Autodesk Inventor part; units mm, degrees
ref_plane "YZ Plane" through (0, 0, 0) normal (1, 0, 0) x (0, 1, 0)
ref_plane "XZ Plane" through (0, 0, 0) normal (0, 1, 0) x (-1, 0, 0)
ref_plane "XY Plane" through (0, 0, 0) normal (0, 0, 1) x (1, 0, 0)
sketch "Sketch1" plane through (0, 0, 0) normal (0, 1, 0) x (-1, 0, 0)
  circle A0 centre (0, 0) radius 4
  line L0 (4, 0) -> (5, 0) construction
  line L1 (5, 0) -> (5, -0.5)
  line L2 (5, -0.5) -> (3.8219, -1.1802)
  line L3 (5, 0) -> (5, 0.5)
  line L4 (5, 0.5) -> (3.8219, 1.1802)
  line L5 (3.8891, 3.182) -> (3.537, 1.868)
  line L6 (3.5355, 3.5355) -> (3.8891, 3.182)
  line L7 (3.5355, 3.5355) -> (3.182, 3.8891)
  line L8 (3.182, 3.8891) -> (1.868, 3.537)
  line L9 (0.5, 5) -> (1.1802, 3.8219)
  line L10 (0, 5) -> (0.5, 5)
  line L11 (0, 5) -> (-0.5, 5)
  line L12 (-0.5, 5) -> (-1.1802, 3.8219)
  line L13 (-3.182, 3.8891) -> (-1.868, 3.537)
  line L14 (-3.5355, 3.5355) -> (-3.182, 3.8891)
  line L15 (-3.5355, 3.5355) -> (-3.8891, 3.182)
  line L16 (-3.8891, 3.182) -> (-3.537, 1.868)
  line L17 (-5, 0.5) -> (-3.8219, 1.1802)
  line L18 (-5, 0) -> (-5, 0.5)
  line L19 (-5, 0) -> (-5, -0.5)
  line L20 (-5, -0.5) -> (-3.8219, -1.1802)
  line L21 (-3.8891, -3.182) -> (-3.537, -1.868)
  line L22 (-3.5355, -3.5355) -> (-3.8891, -3.182)
  line L23 (-3.5355, -3.5355) -> (-3.182, -3.8891)
  line L24 (-3.182, -3.8891) -> (-1.868, -3.537)
  line L25 (-0.5, -5) -> (-1.1802, -3.8219)
  line L26 (0, -5) -> (-0.5, -5)
  line L27 (0, -5) -> (0.5, -5)
  line L28 (0.5, -5) -> (1.1802, -3.8219)
  line L29 (3.182, -3.8891) -> (1.868, -3.537)
  line L30 (3.5355, -3.5355) -> (3.182, -3.8891)
  line L31 (3.5355, -3.5355) -> (3.8891, -3.182)
  line L32 (3.8891, -3.182) -> (3.537, -1.868)
  circle A1 centre (0, 0) radius 17.5 construction
  arc A2 (15.5, -2) -> (15.5, 2) centre (15.5, 0) ccw
  line L33 (15.5, 2) -> (0, 2) construction
  line L34 (15.5, -2) -> (0, -2) construction
  line L35 (16.0176, 1.9319) -> (5.8875, 4.6462)
  line L36 (20.0758, 0) -> (0, 0) construction
  line L37 (16.0176, -1.9319) -> (5.8875, -4.6462)
  line L38 (-1.9319, 16.0176) -> (-4.6462, 5.8875)
  line L39 (1.9319, 16.0176) -> (4.6462, 5.8875)
  arc A3 (2, 15.5) -> (-2, 15.5) centre (0, 15.5) ccw
  line L40 (-16.0176, -1.9319) -> (-5.8875, -4.6462)
  line L41 (-16.0176, 1.9319) -> (-5.8875, 4.6462)
  arc A4 (-15.5, 2) -> (-15.5, -2) centre (-15.5, 0) ccw
  line L42 (1.9319, -16.0176) -> (4.6462, -5.8875)
  line L43 (-1.9319, -16.0176) -> (-4.6462, -5.8875)
  arc A5 (-2, -15.5) -> (2, -15.5) centre (0, -15.5) ccw
  arc A6 (5.8875, 4.6462) -> (4.6462, 5.8875) centre (0, 0) ccw
  arc A7 (-4.6462, 5.8875) -> (-5.8875, 4.6462) centre (0, 0) ccw
  arc A8 (-5.8875, -4.6462) -> (-4.6462, -5.8875) centre (0, 0) ccw
  arc A9 (4.6462, -5.8875) -> (5.8875, -4.6462) centre (0, 0) ccw
  circle A10 centre (0, 15.5) radius 1.25
  circle A11 centre (0, 9.5) radius 1.25
  circle A12 centre (-9.5, 0) radius 1.25
  circle A13 centre (-15.5, 0) radius 1.25
  circle A14 centre (0, -9.5) radius 1.25
  circle A15 centre (0, -15.5) radius 1.25
  circle A16 centre (9.5, 0) radius 1.25
  circle A17 centre (15.5, 0) radius 1.25
  point P0 (-3.8219, -1.1802)
  point P1 (-3.8219, 1.1802)
  dimension "d0" = 8
  dimension "d1" = 120
  dimension "d2" = 1
  dimension "d3" = 0.5
  dimension "d4" = 5
  dimension "d7" = 360
  dimension "d9" = 35
  dimension "d11" = 4
  dimension "d14" = 15
  dimension "d15" = 0
  dimension "d18" = 360
  dimension "d20" = 7.5
  dimension "d21" = 0.8157
  dimension "d22" = 4.0798
  dimension "d23" = 7.9436
  dimension "d24" = 2.5
  dimension "d25" = 2.5
  dimension "d26" = 6
  dimension "d27" = 9.5
  dimension "d30" = 360
extrude "Extrusion1" add sketch "Sketch1" along normal mid plane 8
thread "Thread1"
thread "Thread2"
thread "Thread3"
thread "Thread4"
thread "Thread5"
thread "Thread6"
thread "Thread7"
thread "Thread8"
thread "Thread9"
properties part number "servo horn" material "Titanium"
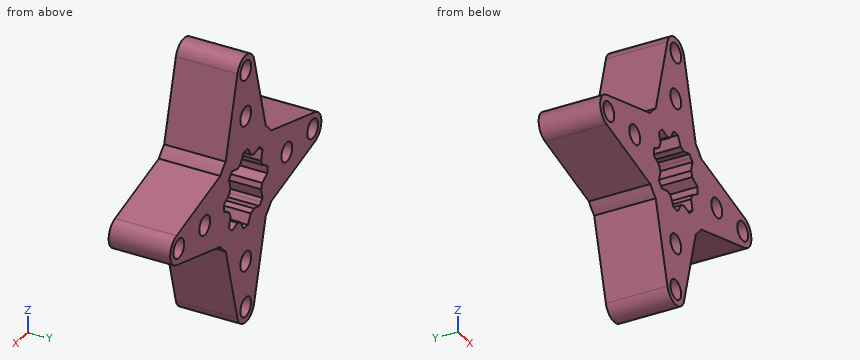
Can you work these out from the model? Positions are in its coordinate system, mm. Round coordinates to 2 decimals unless told otherwise and drop trailing zeros. Write each loop counter-clockwise with the first axis right and the second up, starting at its lowest first coordinate (ties: lowest second). Pieces come first, ordered by that corner, then holes. Notation, with made-up numbers: (78.25, 59.5) -> (120.25, 59.5) arc R23 cw to (120.25, 79.5) -> close; hole circle Ø3 at (57, 27.5). An arc over 180 degrees is marked (long way). One line per question, with ' | ' between items. Start each with the question number.
1) Suppose I cut it at B-B on x = 0. Write out the boundary of the cut face in (y, z).
2) Suppose I cut it at A-A on z = 0. Write out the boundary of the cut face in (x, y).
3) I need wall thicknesses on line 1 (Z direction, x = 15, y = -1.5); line 2 (Z direction, x = -9.5, y = 0.75); line 3 (X direction, y = -3.5, z = -10). Which ranges of each line are inside material? Lowest first, please. Write a range as [from, to].
4) Suppose I cut it at C-C on z = -9.5. Write out the boundary of the cut face in (x, y), then the cut area to 3 significant figures.
5) I'm going to push flat-ended pins straight in: P1, Ø3, axis at x = 0, z = 9.5, coming from the +Y side; P2, Ø1, axis at y = 1.5, z = 13, coming from the +X side; P3, Ø1, axis at x = 12.5, y = -1, coming from the +Z side. Where does each tip first touch, or does it pass through?
6) Suppose I cut it at D-D on x = 15.5. Write out the boundary of the cut face in (y, z).
Return value:
1) outline: (-4, -17.5) -> (4, -17.5) -> (4, -16.75) -> (-4, -16.75) -> close; (-4, -14.25) -> (4, -14.25) -> (4, -10.75) -> (-4, -10.75) -> close; (-4, -8.25) -> (4, -8.25) -> (4, -5) -> (-4, -5) -> close; (-4, 5) -> (4, 5) -> (4, 8.25) -> (-4, 8.25) -> close; (-4, 10.75) -> (4, 10.75) -> (4, 14.25) -> (-4, 14.25) -> close; (-4, 16.75) -> (4, 16.75) -> (4, 17.5) -> (-4, 17.5) -> close
2) outline: (-17.5, -4) -> (-16.75, -4) -> (-16.75, 4) -> (-17.5, 4) -> close; (-14.25, -4) -> (-10.75, -4) -> (-10.75, 4) -> (-14.25, 4) -> close; (-8.25, -4) -> (-5, -4) -> (-5, 4) -> (-8.25, 4) -> close; (5, -4) -> (8.25, -4) -> (8.25, 4) -> (5, 4) -> close; (10.75, -4) -> (14.25, -4) -> (14.25, 4) -> (10.75, 4) -> close; (16.75, -4) -> (17.5, -4) -> (17.5, 4) -> (16.75, 4) -> close
3) line 1: z = [-2.2, -1.15], [1.15, 2.2] | line 2: z = [-3.68, -1.25], [1.25, 3.68] | line 3: x = [-3.54, -1.15], [1.15, 3.54]
4) outline: (-3.68, -4) -> (-1.25, -4) -> (-1.25, 4) -> (-3.68, 4) -> close; (1.25, -4) -> (3.68, -4) -> (3.68, 4) -> (1.25, 4) -> close | area: 38.9 mm2
5) P1: stops at y = 4 | P2: stops at x = 2.87 | P3: stops at z = 3.01
6) outline: (-4, -2.07) -> (4, -2.07) -> (4, -1.25) -> (-4, -1.25) -> close; (-4, 1.25) -> (4, 1.25) -> (4, 2.07) -> (-4, 2.07) -> close
